```python
from build123d import *

# Parameters (mm, degrees)
SKETCH074_W             = 30
SKETCH074_H             = 62
PAD034_DEPTH            = 4
PAD084_DEPTH            = 20
SKETCH164_R             = 1.55
POCKET003_DEPTH         = 5
CHAMFER_SIZE            = 3
FILLET_R                = 3
FILLET001_R             = 5
SKETCH_R                = 1.375
POCKET_DEPTH            = 19.001
POCKET_DEPTH_BACK       = -11.001
SKETCH166_R             = 2.95
POCKET004_DEPTH         = 5
SKETCH167_R             = 1.55
POCKET005_DEPTH         = 2.5
SKETCH168_R             = 3
POCKET006_DEPTH         = 5
BODY010_PITCH_ANGLE     = 90
BODY010_PLACEMENT_ANGLE = -180


with BuildPart() as part:
    # Sketch074 → Pad034 (new body)
    with BuildSketch(Plane.XZ):
        with Locations((15, -16)):
            Rectangle(SKETCH074_W, SKETCH074_H)
    extrude(amount=PAD034_DEPTH)

    # Sketch160 (on Face3 of Pad034) → Pad084 (join)
    with BuildSketch(Plane(origin=(0, 0, -47), x_dir=(1, 0, 0), z_dir=(0, 0, -1))):
        with BuildLine():
            Line((0, 0), (0, 19))
            ThreePointArc((11, 33.456832), (3.062664, 28.082951), (0, 19))
            Line((11, 38.456832), (11, 33.456832))
            Line((13.5, 38.456832), (11, 38.456832))
            Line((13.5, 31.30894), (13.5, 38.456832))
            ThreePointArc((13.5, 31.30894), (15, 6.6), (16.5, 31.30894))
            Line((16.5, 31.30894), (16.5, 38.456832))
            Line((16.5, 38.456832), (19, 38.456832))
            Line((19, 38.456832), (19, 33.456832))
            ThreePointArc((30, 19), (26.937336, 28.082951), (19, 33.456832))
            Line((30, 19), (30, 0))
            Line((30, 0), (0, 0))
        make_face()
    extrude(amount=-PAD084_DEPTH)

    # Sketch164 → Pocket003 (cut)
    with BuildSketch(Plane.XZ.offset(4)):
        with Locations((8.504809, 7.5)):
            Circle(SKETCH164_R)
        with Locations((8.504809, -7.5)):
            Circle(SKETCH164_R)
        with Locations((21.495191, 0)):
            Circle(SKETCH164_R)
        with Locations((15, 11.5)):
            Circle(SKETCH164_R)
    extrude(amount=-POCKET003_DEPTH, mode=Mode.SUBTRACT)

    # Sketch165 (on DatumPlane) → Groove (revolve, cut)
    with BuildSketch(Plane(origin=(15, 0, 0), x_dir=(0, 0, 1), z_dir=(1, 0, 0))):
        with BuildLine():
            Line((-51.816792, 23.505394), (-59.215083, 23.505394))
            Line((-59.215083, 23.505394), (-59.215083, 49.506645))
            Line((-59.215083, 49.506645), (-28.913541, 49.506645))
            Line((-28.913541, 49.506645), (-28.913541, 43.218523))
            ThreePointArc((-28.913541, 43.218523), (-42.969663, 36.387934), (-51.816792, 23.505394))
        make_face()
    revolve(axis=Axis((15, -19, 0), (0, 0, 1)), mode=Mode.SUBTRACT)

    # Chamfer
    chamfer_edges = [part.edges().sort_by_distance(p)[0] for p in [
        (17.75, -38.456832, -27),
        (12.25, -38.456832, -27),
    ]]
    chamfer(chamfer_edges, length=CHAMFER_SIZE)

    # Fillet
    fillet_edges = [part.edges().sort_by_distance(p)[0] for p in [
        (15, -4, -27),
    ]]
    fillet(fillet_edges, radius=FILLET_R)

    # Fillet001
    fillet001_edges = [part.edges().sort_by_distance(p)[0] for p in [
        (11, -33.456832, -36.223655),
        (19, -33.456832, -36.223655),
    ]]
    fillet(fillet001_edges, radius=FILLET001_R)

    # Sketch (on Face10 of Fillet001) → Pocket (cut, two sides)
    with BuildSketch(Plane(origin=(19, 0, 0), x_dir=(0, 0, 1), z_dir=(1, 0, 0))) as pocket_sk:
        with Locations((-35, 35)):
            Circle(SKETCH_R)
    extrude(amount=-POCKET_DEPTH, mode=Mode.SUBTRACT)
    extrude(pocket_sk.sketch, amount=-POCKET_DEPTH_BACK, mode=Mode.SUBTRACT)

    # Sketch166 (on Face10 of Pocket) → Pocket004 (cut)
    with BuildSketch(Plane(origin=(19, 0, 0), x_dir=(0, 0, 1), z_dir=(1, 0, 0))):
        with Locations((-35, 35)):
            Circle(SKETCH166_R)
    extrude(amount=POCKET004_DEPTH, mode=Mode.SUBTRACT)

    # Sketch167 (on Face23 of Pocket004) → Pocket005 (cut)
    with BuildSketch(Plane(origin=(19, 0, 0), x_dir=(0, 0, 1), z_dir=(1, 0, 0))):
        with Locations((-35, 35)):
            Circle(SKETCH167_R)
    extrude(amount=-POCKET005_DEPTH, mode=Mode.SUBTRACT)

    # Sketch168 (on Face17 of Pocket005) → Pocket006 (cut)
    with BuildSketch(Plane.XZ.offset(4)):
        with Locations((15, 0)):
            Circle(SKETCH168_R)
    extrude(amount=-POCKET006_DEPTH, mode=Mode.SUBTRACT)


with BuildPart() as part_1:
    # Body010 pitch: moved
    add(part.part.rotate(Axis((0, 0, 0), (0, 1, 0)), BODY010_PITCH_ANGLE))


with BuildPart() as part_2:
    # Body010 placement: moved
    add(part_1.part.rotate(Axis((0, 0, 0), (0, 0, 1)), BODY010_PLACEMENT_ANGLE))


solid = part_2.part
```
The listing builds one solid part. Answer for the finished solid, in the listing's coordinates (mm). A direction names the side the tool comes from. Give positions to 0.01 mm unless a question says otherwise; leave off trailing zeros. Loops run counter-clockwise (first coordinate to the right, second up) from the corner with the lowest first, then second, coordinate; pieces in that order, holes last. Notation, with made-up numbers: (-24, 75) - (-5, 75) arc R21 cw to (-5, 90) - close; hole circle Ø3 at (86.5, 45). An arc over 180 degrees is marked (long way). Return JSON: item names as keys, results as strings. Group by question number.
1. Find section B-B (x = -11.5). Write down the section's boundary in (y, z), then the cut area to 3 significant figures.
2. Find section D-D (x = 17). Write down the section's boundary in (y, z), then the cut area to 3 significant figures.
3. Determine the mould class of faces 1 (the cylindrical face through (35.336, 33.487, -17.768)), 2 (the cylindrical face through (35.3, 33.66, -12.09)), 3 (the flat face through (37, 34, -16.5)), 4 (the flat face through (28.521, 36.978, -17.832)) for opening direction X: pulls with the +X half, pulls with the -X half, needs draft (parallel to the pull), parting line crosses it, or undercut.
4. Find section A-A (x = 0). Write down the section's boundary in (y, z), then the cut area to 3 significant figures.
5. Straight lines are drawn through the part: line 1 (Z direction, x = 0, y = 1); line 2 (Y direction, x = 35, z = -18); line 3 (Z direction, x = -11.5, y = 1.85). For each, find the intervals that lie inside material, in ascending order. Write a range as [from, to].
6. Find section C-C (z = -15). State how many separate pieces and enclosed holes the cut face has, then the cut area to 3 significant figures.
7. Given pin 1 Ø1.3 at (x, y) = (33.5, 38) entering from +Z; pin 2 Ø4 at (x, z) = (-7.5, -8.5) entering from +Y; pin 3 Ø11 at (y, z) = (16.5, -10) entering from -X; pin 4 Ø3.5 at (x, y) = (37.5, 34) entering from -Z, each flat-ended and moving along its own axis, determine where each tip first touches the part or whether it passes through.
8. Which of the six approach directions +Z, -Z, +X, -X, +Y, -Y give full straight-line access (tool end or side, diameter ignored) to faces 5 (the flat face through (27, 19, -2)), 6 (the flat face through (35, 38.457, -18)), 7 (the flat face through (35, 38, -11))?
Verdict:
{
 "1": {"outline": "(0, -30) - (4, -30) - (4, -16.55) - (0, -16.55) - close; (0, -13.45) - (4, -13.45) - (4, 0) - (0, 0) - close", "area": "108 mm^2"},
 "2": {"outline": "(0, -30) - (4, -30) - (4, 0) - (0, 0) - close", "area": "120 mm^2"},
 "3": {"face 1": "undercut", "face 2": "undercut", "face 3": "needs draft", "face 4": "pulls with the -X half"},
 "4": {"outline": "(0, -30) - (4, -30) - (4, -23.05) - (0, -23.05) - close; (0, -19.95) - (4, -19.95) - (4, -18) - (0, -18) - close; (0, -12) - (4, -12) - (4, 0) - (0, 0) - close", "area": "83.6 mm^2"},
 "5": {"line 1": "z = [-30, -23.05], [-19.95, -18], [-12, 0]", "line 2": "y = [0, 6.97], [31.03, 33.45], [36.55, 38.46]", "line 3": "z = [-30, -16.55], [-13.45, 0]"},
 "6": {"separate pieces": "3", "enclosed holes": "0", "area": "249 mm^2"},
 "7": {"pin 1": "stops at z = -11", "pin 2": "stops at y = 4", "pin 3": "passes through", "pin 4": "stops at z = -22.03"},
 "8": {"face 5": "+Z, -Z, -X, +Y", "face 6": "+Z, -Z, +X, -X, +Y", "face 7": "+Z, +X, -X, +Y"}
}
